```python
from build123d import *

# Parameters (mm, degrees)
SKETCH1_W                         = 283
SKETCH1_H                         = 225
SKETCH1_W_2                       = 258
SKETCH1_H_2                       = 200
WALLS_DEPTH                       = 90
SKETCH3_W                         = 283
SKETCH3_H                         = 225
BASE_DEPTH                        = 12.5
SKETCH4_W                         = 12
SKETCH4_H                         = 15.1
LONG_SUPPORT_DEPTH                = 114.5
SKETCH5_W                         = 12
SKETCH5_H                         = 15.1
SHORT_SUPPORT_DEPTH               = 25
RESERVOIR_OUTFLOW_TUBE_HOLE_REACH = 359.065
SKETCH6_R                         = 6.35
SKETCH7_W                         = 101
SKETCH7_H                         = 26
CONNECTOR_PORT_SHORTSIDE_DEPTH    = 283
LPATTERN1_COUNT                   = 2
LPATTERN1_PITCH                   = 270.5
SKETCH8_W                         = 101
SKETCH8_H                         = 26
CONNECTOR_PORT_LONGSIDE_DEPTH     = 225
LPATTERN2_COUNT                   = 2
LPATTERN2_PITCH                   = 212.5
SKETCH9_W                         = 283
SKETCH9_H                         = 225
SKETCH9_W_2                       = 258
SKETCH9_H_2                       = 200
LOWER_WATER_JACKET_WALLS_DEPTH    = 50
SKETCH11_W                        = 283
SKETCH11_H                        = 225
LOWER_WATER_JACKET_BOTTOM_DEPTH   = 12.5


with BuildPart() as part:
    # Sketch1 → Walls (new body)
    with BuildSketch(Plane(origin=(0, 0, 0), x_dir=(1, 0, 0), z_dir=(0, 1, 0))):
        with Locations((126.5, 102.5)):
            Rectangle(SKETCH1_W, SKETCH1_H)
        with Locations((126.5, 102.5)):
            Rectangle(SKETCH1_W_2, SKETCH1_H_2, mode=Mode.SUBTRACT)
    extrude(amount=WALLS_DEPTH)

    # Sketch3 → Base (add)
    with BuildSketch(Plane.XZ):
        with Locations((126.5, -102.5)):
            Rectangle(SKETCH3_W, SKETCH3_H)
    extrude(amount=BASE_DEPTH)

    # Sketch4 → Long_Support (add, symmetric)
    with BuildSketch(Plane(origin=(126.5, 0, 0), x_dir=(0, 0, -1), z_dir=(1, 0, 0))):
        with Locations((8.5, 42.45)):
            Rectangle(SKETCH4_W, SKETCH4_H)
        with Locations((196.5, 42.45)):
            Rectangle(SKETCH4_W, SKETCH4_H)
    extrude(amount=LONG_SUPPORT_DEPTH, both=True)

    # Sketch5 → Short_Support (add, symmetric)
    with BuildSketch(Plane(origin=(0, 0, -102.5), x_dir=(-1, 0, 0), z_dir=(0, 0, -1))):
        with Locations((-249.5, 42.45)):
            Rectangle(SKETCH5_W, SKETCH5_H)
        with Locations((-3.5, 42.45)):
            Rectangle(SKETCH5_W, SKETCH5_H)
    extrude(amount=SHORT_SUPPORT_DEPTH, both=True)

    # Sketch6 → Reservoir_Outflow_Tube_Hole (cut, up to next)
    with BuildSketch(Plane(origin=(-2.5, 0, 0), x_dir=(0, 0, -1), z_dir=(1, 0, 0)), mode=Mode.PRIVATE) as reservoir_outflow_tube_hole_sk1:
        with Locations((171.15, 43.65)):
            Circle(SKETCH6_R)
    reservoir_outflow_tube_hole_tool1 = extrude(reservoir_outflow_tube_hole_sk1.sketch, amount=-RESERVOIR_OUTFLOW_TUBE_HOLE_REACH, mode=Mode.PRIVATE) & part.part
    add(reservoir_outflow_tube_hole_tool1.solids().sort_by_distance((-2.5, 43.65, -171.15))[0], mode=Mode.SUBTRACT)

    # Sketch7 → Connector_Port_ShortSide (cut)
    with BuildSketch(Plane(origin=(-2.5, 0, 0), x_dir=(0, 0, -1), z_dir=(1, 0, 0))):
        with Locations((102.5, 67)):
            Rectangle(SKETCH7_W, SKETCH7_H)
    connector_port_shortside = extrude(amount=-CONNECTOR_PORT_SHORTSIDE_DEPTH, mode=Mode.SUBTRACT)

    # LPattern1: Connector_Port_ShortSide ×2
    with Locations(*[(i * LPATTERN1_PITCH, 0, 0) for i in range(1, LPATTERN1_COUNT)]):
        add(connector_port_shortside, mode=Mode.SUBTRACT)

    # Sketch8 → Connector_Port_LongSide (cut)
    with BuildSketch(Plane.XY.offset(-2.5)):
        with Locations((126.5, 67)):
            Rectangle(SKETCH8_W, SKETCH8_H)
    connector_port_longside = extrude(amount=CONNECTOR_PORT_LONGSIDE_DEPTH, mode=Mode.SUBTRACT)

    # LPattern2: Connector_Port_LongSide ×2
    with Locations(*[(0, 0, -i * LPATTERN2_PITCH) for i in range(1, LPATTERN2_COUNT)]):
        add(connector_port_longside, mode=Mode.SUBTRACT)

    # Sketch9 → Lower_Water_Jacket_Walls (add)
    with BuildSketch(Plane.XZ.offset(12.5)):
        with Locations((126.5, -102.5)):
            Rectangle(SKETCH9_W, SKETCH9_H)
        with Locations((126.5, -102.5)):
            Rectangle(SKETCH9_W_2, SKETCH9_H_2, mode=Mode.SUBTRACT)
    extrude(amount=LOWER_WATER_JACKET_WALLS_DEPTH)

    # Sketch11 → Lower_Water_Jacket_Bottom (add)
    with BuildSketch(Plane.XZ.offset(62.5)):
        with Locations((126.5, -102.5)):
            Rectangle(SKETCH11_W, SKETCH11_H)
    extrude(amount=LOWER_WATER_JACKET_BOTTOM_DEPTH)


solid = part.part
```
Source: CAD feature listing. Evaluate the final solid. Frame: model axes, mm. A direction names the side the tool comes from. Coordinates: 2 decimals unless noted, no trailing zeros. Loops run counter-clockwise (first coordinate to the right, second up) from the corner with the lowest first, then second, coordinate; pieces in that order, holes last. Notation, with made-up numbers: M 83,-38 L 124,-38 A27 cw 124,-1 Z; hole C -18.5,28.25 d5. An arc over 180 degrees is marked long. Use a Markdown table: item, result. Add a question column.
Q1. Section query A-A, the plane x = 129.5. Return loops of the section in (y, z).
Q2. Access query for faces 3 (the flat face through (177, 67, 4)), 4 (the flat face through (243.5, 42, -102)), 5 (the flat face through (255.5, -37, -104)). Directions: +Z, -Z, +X, -X, +Y, -Y. A direction counts if a zero-diameter tool reaches every point of the face in a straight line with its end or side. Return the directions, or none.
Q3. Material intervals for L1, parallel to Y at x = 44, z = -196.5; L2, parallel to Z at x = 64, y = -62; L3, parallel to X at y = 1, z = -24, sorted ascending.
Q4. Draft query along X for faces 1 (the flat face through (128, 50, -196)), 2 (the flat face through (268, 9, -104)). Return one class per face: pulls with the +X half, pulls with the -X half, needs draft (parallel to the pull), parting line crosses it, or undercut.
Q5. Section query D-D, the plane y = 68. Return loops of the section in (x, z), and give its area (4 significant figures).
Q6. Section query C-C, the plane z = -118.5. Return loops of the section in (x, y).
Q7. Section query B-B, the plane z = -198. Return loops of the section in (x, y), and give its area (3 significant figures).
Result:
| question | item | result |
|---|---|---|
| 1 | outline | M -75,-215 L 54,-215 L 54,-202.5 L 50,-202.5 L 50,-190.5 L 34.9,-190.5 L 34.9,-202.5 L 0,-202.5 L 0,-2.5 L 34.9,-2.5 L 34.9,-14.5 L 50,-14.5 L 50,-2.5 L 54,-2.5 L 54,10 L -75,10 Z; M 80,-215 L 90,-215 L 90,-202.5 L 80,-202.5 Z; M 80,-2.5 L 90,-2.5 L 90,10 L 80,10 Z; hole M -62.5,-202.5 L -12.5,-202.5 L -12.5,-2.5 L -62.5,-2.5 Z |
| 2 | face 3 | +Z, -Z |
| 2 | face 4 | +Y |
| 2 | face 5 | none |
| 3 | L1 | y = -75 to -62.5, -12.5 to 0, 34.9 to 50 |
| 3 | L2 | z = -215 to -202.5, -2.5 to 10 |
| 3 | L3 | x = -15 to -2.5, 255.5 to 268 |
| 4 | face 1 | undercut |
| 4 | face 2 | pulls with the +X half |
| 5 | outline | M -15,-215 L 76,-215 L 76,-202.5 L -2.5,-202.5 L -2.5,-153 L -15,-153 Z; M -15,-52 L -2.5,-52 L -2.5,-2.5 L 76,-2.5 L 76,10 L -15,10 Z; M 177,-215 L 268,-215 L 268,-153 L 255.5,-153 L 255.5,-202.5 L 177,-202.5 Z; M 177,-2.5 L 255.5,-2.5 L 255.5,-52 L 268,-52 L 268,10 L 177,10 Z |
| 5 | area | 7,025 mm2 |
| 6 | outline | M -15,-75 L 268,-75 L 268,54 L 255.5,54 L 255.5,50 L 243.5,50 L 243.5,34.9 L 255.5,34.9 L 255.5,0 L -2.5,0 L -2.5,34.9 L 9.5,34.9 L 9.5,50 L -2.5,50 L -2.5,54 L -15,54 Z; M -15,80 L -2.5,80 L -2.5,90 L -15,90 Z; M 255.5,80 L 268,80 L 268,90 L 255.5,90 Z; hole M -2.5,-62.5 L 255.5,-62.5 L 255.5,-12.5 L -2.5,-12.5 Z |
| 7 | outline | M -15,-75 L 268,-75 L 268,90 L 255.5,90 L 255.5,0 L -2.5,0 L -2.5,90 L -15,90 Z; M 12,34.9 L 241,34.9 L 241,50 L 12,50 Z; hole M -2.5,-62.5 L 255.5,-62.5 L 255.5,-12.5 L -2.5,-12.5 Z |
| 7 | area | 14,000 mm2 |
